Geometry: final body of the model. Coordinates: model frame, mm. Face numbers are marked on the shaded views. Give positions to 0.01 mm unless a question says otherwise; leave off trailing zeros. Loops run counter-clockwise (first coordinate to the right, second up) from the corner with the lowest first, then second, coordinate; pieces in that order, holes last. Notation, with made-up numbers: (-3.75, -13.5) - (29.25, -13.5) arc R13 cw to (29.25, -5.5) - close; hole circle Ø11 at (44.25, 37.5). An arc over 180 degrees is marked (long way). Answer in a Markdown table with one row per item.
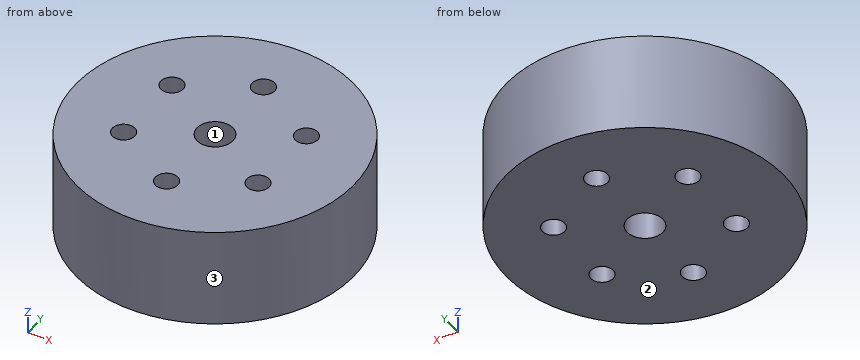
from build123d import *

# Parameters (mm, degrees)
SKETCH1_R           = 15.5
BOSS_EXTRUDE1_DEPTH = 11
SKETCH2_R           = 2
SKETCH2_R_2         = 1.25
CUT_EXTRUDE1_DEPTH  = 11


with BuildPart() as part:
    # Sketch1 → Boss-Extrude1 (new body)
    with BuildSketch(Plane.XY):
        Circle(SKETCH1_R)
    extrude(amount=BOSS_EXTRUDE1_DEPTH)

    # Sketch2 → Cut-Extrude1 (cut)
    with BuildSketch(Plane.XY.offset(11)):
        Circle(SKETCH2_R)
        with Locations((7.555298175, 4.413611842)):
            Circle(SKETCH2_R_2)
        with Locations((7.555079083, -4.336388156)):
            Circle(SKETCH2_R_2)
        with Locations((-0.022752744, -8.711198415)):
            Circle(SKETCH2_R_2)
        with Locations((-7.600365479, -4.336008677)):
            Circle(SKETCH2_R_2)
        with Locations((-7.600146387, 4.413991321)):
            Circle(SKETCH2_R_2)
        with Locations((-0.02231456, 8.78880158)):
            Circle(SKETCH2_R_2)
    extrude(amount=-CUT_EXTRUDE1_DEPTH, mode=Mode.SUBTRACT)


solid = part.part
Q1. Cut plane D-D (y = -8). Output: boundary loops of the cut face in (x, z).
Check values:
| item | result |
|---|---|
| outline | (-13.28, 0) - (-1.05, 0) - (-1.05, 11) - (-13.28, 11) - close; (1.01, 0) - (13.28, 0) - (13.28, 11) - (1.01, 11) - close |
Q2. Cut plane B-B (x = -0.5). Output: boundary loops of the cut face in (y, z).
Check values:
| item | result |
|---|---|
| outline | (-15.49, 0) - (-9.87, 0) - (-9.87, 11) - (-15.49, 11) - close; (-7.56, 0) - (-1.94, 0) - (-1.94, 11) - (-7.56, 11) - close; (1.94, 0) - (7.63, 0) - (7.63, 11) - (1.94, 11) - close; (9.94, 0) - (15.49, 0) - (15.49, 11) - (9.94, 11) - close |
Q3. Cut plane C-C (z = 2.5). Output: boundary loops of the cut face in (x, y), and give its area (3 significant figures).
Check values:
| item | result |
|---|---|
| outline | circle Ø31 at (0, 0); hole circle Ø2.5 at (-7.6, -4.34); hole circle Ø2.5 at (-7.6, 4.41); hole circle Ø4 at (0, 0); hole circle Ø2.5 at (-0.02, -8.71); hole circle Ø2.5 at (-0.02, 8.79); hole circle Ø2.5 at (7.56, -4.34); hole circle Ø2.5 at (7.56, 4.41) |
| area | 713 mm² |
Q4. Draft query along X for the marked faces 1, 2 and 3. Return one class per face: pulls with the +X half, pulls with the -X half, needs draft (parallel to the pull), parting line crosses it, or undercut.
Check values:
| item | result |
|---|---|
| face 1 | undercut |
| face 2 | needs draft |
| face 3 | parting line crosses it |
Q5. Material intervals for line 1 along Y through (x, z) = (0.5, 5.5); line 2 along X through (y, z) = (5.5, 1.5); line 3 along Y through (x, z) = (8, 8.5), sorted ascending.
Check values:
| item | result |
|---|---|
| line 1 | -15.49 to -9.85, -7.58 to -1.94, 1.94 to 7.65, 9.92 to 15.49 |
| line 2 | -14.49 to -8.22, -6.98 to 6.94, 8.17 to 14.49 |
| line 3 | -13.28 to -5.5, -3.17 to 3.25, 5.58 to 13.28 |
Q6. Cut plane A-A (y = 0). Output: boundary loops of the cut face in (x, z), and give its area (3 significant figures).
Check values:
| item | result |
|---|---|
| outline | (-15.5, 0) - (-2, 0) - (-2, 11) - (-15.5, 11) - close; (2, 0) - (15.5, 0) - (15.5, 11) - (2, 11) - close |
| area | 297 mm² |
Q7. First-contact query: pin 1 (1 mm diameter, centred on x = 11.5, z = 8.5, fed in from -Y); pin 2 (1.5 mm diameter, centred on x = -0.02, y = 8.79, fed in from -Z); pin 3 (3 mm diameter, centred on x = -7.6, y = -4.34, fed in from +Z); pin 4 (5 mm diameter, centred on x = 5, z = 4, fed in from +Y). Flat tips, straight axial feed; report the tip coordinate or a pass-through.
Check values:
| item | result |
|---|---|
| pin 1 | y = -10.92 |
| pin 2 | through |
| pin 3 | z = 11 |
| pin 4 | y = 15.3 |
